```python
from build123d import *

# Parameters (mm, degrees)
SKETCH1_W           = 66
SKETCH1_H           = 47
SKETCH1_W_2         = 59
SKETCH1_H_2         = 41
BOSS_EXTRUDE1_DEPTH = 10
SKETCH3_W           = 66
SKETCH3_H           = 47
BOSS_EXTRUDE2_DEPTH = 1
SKETCH6_W           = 1
SKETCH6_H           = 41
SKETCH6_W_2         = 0.5
BOSS_EXTRUDE3_DEPTH = 10


with BuildPart() as part:
    # Sketch1 → Boss-Extrude1 (new body)
    with BuildSketch(Plane(origin=(0, 0, 0), x_dir=(1, 0, 0), z_dir=(0, 1, 0))):
        Rectangle(SKETCH1_W, SKETCH1_H)
        Rectangle(SKETCH1_W_2, SKETCH1_H_2, mode=Mode.SUBTRACT)
    extrude(amount=BOSS_EXTRUDE1_DEPTH)

    # Sketch3 → Boss-Extrude2 (add)
    with BuildSketch(Plane(origin=(0, 0, 0), x_dir=(-1, 0, 0), z_dir=(0, -1, 0))):
        Rectangle(SKETCH3_W, SKETCH3_H)
    extrude(amount=BOSS_EXTRUDE2_DEPTH)

    # Sketch6 → Boss-Extrude3 (add)
    with BuildSketch(Plane(origin=(0, 10, 0), x_dir=(1, 0, 0), z_dir=(0, 1, 0))):
        with Locations((-15, 0)):
            Rectangle(SKETCH6_W, SKETCH6_H)
        with Locations((-0.25, 0)):
            Rectangle(SKETCH6_W_2, SKETCH6_H)
        with Locations((0.25, 0)):
            Rectangle(SKETCH6_W_2, SKETCH6_H)
        with Locations((15, 0)):
            Rectangle(SKETCH6_W, SKETCH6_H)
    extrude(amount=-BOSS_EXTRUDE3_DEPTH)


solid = part.part
```
Source: CAD feature listing. Evaluate the final solid. Frame: model axes, mm. A direction names the side the tool comes from. Round coordinates to 2 decimals unless told otherwise and drop trailing zeros. Write each loop counter-clockwise with the first axis right and the second up, starting at its lowest first coordinate (ties: lowest second). Pieces come first, ordered by that corner, then holes. Notation, with made-up numbers: M 76.25,89.25 L 111.25,89.25 A14 ccw 111.25,103.25 Z; hole C -21.5,-18.75 d9. An arc over 180 degrees is marked long. Use CSV: the item, a comma, the result in double quotes. Start each with the question number.
Q1. Pull-direction query (X, two-part tool) for faces 1 (the face through (0, -1, 0)), 2 (the face through (23, 0, 0)); classes: +X half, -X half, draft (parallel to the pull), parting line (faces both ways), or undercut.
Q2. Access query for faces 3 (the face through (7, 5, 20.5)), 4 (the face through (-15, 10, 0)). Directions: +Z, -Z, +X, -X, +Y, -Y. A direction counts if a zero-diameter tool reaches every point of the face in a straight line with its end or side. Return the directions, or none.
Q3. Cut plane B-B on x = -9.5. Output: boundary loops of the cut face in (y, z), plus the area to 3 significant figures.
Q4. First-contact query: P1, Ø3, axis at x = 26, z = -9, coming from the +Y side; P2, Ø15.5, axis at x = -20, z = -3, coming from the +Y side. Flat tips, straight axial feed; report the tip coordinate or a pass-through.
Q5. Line query: line 1 (X direction, y = 0.5, z = 11); line 2 (Z direction, x = 2, y = 7.75); line 3 (Y direction, x = -12, z = -2). Output: solid intervals per line, ascending. Write a range as from..to.
Q6. Cut plane A-A on y = 5. Output: boundary loops of the cut face in (x, z), plus the area to 3 significant figures.
Q7. Cut plane C-C on z = -19.5. Output: boundary loops of the cut face in (x, y).
Results found:
1,face 1,"draft"
1,face 2,"undercut"
2,face 3,"+Y"
2,face 4,"+Z, -Z, +X, -X, +Y"
3,outline,"M -1,-23.5 L 10,-23.5 L 10,-20.5 L 0,-20.5 L 0,20.5 L 10,20.5 L 10,23.5 L -1,23.5 Z"
3,area,"107 mm^2"
4,P1,"y = 0"
4,P2,"y = 10"
5,line 1,"-33..-29.5, -15.5..-14.5, -0.5..0.5, 14.5..15.5, 29.5..33"
5,line 2,"-23.5..-20.5, 20.5..23.5"
5,line 3,"-1..0"
6,outline,"M -33,-23.5 L 33,-23.5 L 33,23.5 L -33,23.5 Z; hole M -29.5,-20.5 L -15.5,-20.5 L -15.5,20.5 L -29.5,20.5 Z; hole M -14.5,-20.5 L -0.5,-20.5 L -0.5,20.5 L -14.5,20.5 Z; hole M 0.5,-20.5 L 14.5,-20.5 L 14.5,20.5 L 0.5,20.5 Z; hole M 15.5,-20.5 L 29.5,-20.5 L 29.5,20.5 L 15.5,20.5 Z"
6,area,"806 mm^2"
7,outline,"M -33,-1 L 33,-1 L 33,10 L 29.5,10 L 29.5,0 L 15.5,0 L 15.5,10 L 14.5,10 L 14.5,0 L 0.5,0 L 0.5,10 L -0.5,10 L -0.5,0 L -14.5,0 L -14.5,10 L -15.5,10 L -15.5,0 L -29.5,0 L -29.5,10 L -33,10 Z"
